from build123d import *

# Parameters (mm, degrees)
F1_DEPTH = 6
F2_D     = 12.5
F3_D     = 5
F4_D     = 5
F5_D     = 5
F6_D     = 5
F7_R     = 5
F8_D     = 8
F8_DEPTH = 20
F8_TIP   = 2.4034424761
F9_D     = 6


with BuildPart() as f1:
    # F0 (on Front) → F1 (new body)
    with BuildSketch(Plane.XZ):
        Polygon((0, 27), (0, -27), (13, -27), (40, -27), (40, 55), (26, 55), (26, 73), (0, 73), align=None)
    extrude(amount=F1_DEPTH)

    # F2 (through all)
    with Locations(Plane(origin=(0, 0, 0), x_dir=(1, 0, 0), z_dir=(0, 1, 0))):
        with Locations((13, 7)):
            Hole(F2_D / 2)

    # F3 (through all)
    with Locations(Plane(origin=(0, 0, 0), x_dir=(1, 0, 0), z_dir=(0, 1, 0))):
        with Locations((34, 21), (34, -32)):
            Hole(F3_D / 2)

    # F4 (through all)
    with Locations(Plane(origin=(0, 0, 0), x_dir=(1, 0, 0), z_dir=(0, 1, 0))):
        with Locations((5, -32), (21, -32)):
            Hole(F4_D / 2)

    # F5 (through all)
    with Locations(Plane(origin=(0, 0, 0), x_dir=(1, 0, 0), z_dir=(0, 1, 0))):
        with Locations((5, 21), (5, -9)):
            Hole(F5_D / 2)

    # F6 (through all)
    with Locations(Plane(origin=(0, 0, 0), x_dir=(1, 0, 0), z_dir=(0, 1, 0))):
        with Locations((5, -68), (21, -68)):
            Hole(F6_D / 2)

    # F7
    f7_edges = [f1.edges().sort_by_distance(p)[0] for p in [
        (26, -3, 73),
        (0, -3, 73),
        (40, -3, 55),
        (26, -3, 55),
        (40, -3, -27),
        (0, -3, -27),
    ]]
    fillet(f7_edges, radius=F7_R)

    # F8
    with Locations(Plane(origin=(0, 0, 0), x_dir=(1, 0, 0), z_dir=(0, 1, 0))):
        with Locations((13, -55.5)):
            Hole(F8_D / 2, depth=F8_DEPTH)
            with Locations((0, 0, -(F8_DEPTH + F8_TIP / 2))):  # 118° drill point
                Cone(0, F8_D / 2, F8_TIP, mode=Mode.SUBTRACT)

    # F9 (through all)
    with Locations(Plane(origin=(0, 0, 0), x_dir=(1, 0, 0), z_dir=(0, 1, 0))):
        with Locations((34, -49)):
            Hole(F9_D / 2)


solid = f1.part
Could you check a few things on this model? Use its own coordinates, in mm. Give positions to 0.01 mm unless a question says otherwise; leave off trailing zeros. Order: outer loops, then holes, each group sorted by start corner. A loop starts at its lowest first (then second) coordinate and runs counter-clockwise, first axis right, second up. Notation, with made-up numbers: (33.25, 17) - (57.25, 17) arc R29 ccw to (57.25, 45) - close; hole circle Ø3 at (-5, -12). An arc over 180 degrees is marked (long way). Return JSON: item names as keys, results as strings. Group by question number.
Q1. Please list where these lines run through material, in increasing order: line 1 along Z through (x, y) = (21, -4.55); line 2 along X through (y, z) = (-2.2, 32); line 3 along Z through (x, y) = (5, -4.3). Write a range as [from, to].
Q2. Will this pin go through, and if not, where does the flat tip stop? pin 1 Ø5 at (x, z) = (12.5, 7.5) entering from +Y.
Q3. Thinking about a two-plate mould opening in X: for faces 1 (the face through (26, -3, 64)), 2 (the face through (3.85, -3.04, 11.22)), 3 (the face through (33, -3, 55)), 4 (the face through (36.21, -3.04, 46.97)), which applies, pulls with the +X half, pulls with the -X half, needs draft (parallel to the pull), parting line crosses it, or undercut?
Q4. Suppose I cut it at A-A, the plane x = 13. Please give me the cut outline in (y, z), and give its area (3 significant figures).
Q5. Suppose I cut it at C-C, the plane z = 9. Please give me the cut outline in (x, y).
Q6. Suppose I cut it at B-B, the plane z = 32. Please give me the cut outline in (x, y), and give its area (3 significant figures).
Q7. Suppose I cut it at D-D, the plane z = -7. Please give me the cut outline in (x, y).
Resolved:
{
 "1": {"line 1": "z = [-27, 29.5], [34.5, 65.5], [70.5, 73]", "line 2": "x = [0, 2.5], [7.5, 18.5], [23.5, 31.5], [36.5, 40]", "line 3": "z = [-27, -23.5], [-18.5, 6.5], [11.5, 29.5], [34.5, 65.5], [70.5, 73]"},
 "2": {"pin 1": "stops at y = 0"},
 "3": {"face 1": "pulls with the +X half", "face 2": "undercut", "face 3": "needs draft", "face 4": "undercut"},
 "4": {"outline": "(-6, -27) - (0, -27) - (0, -13.25) - (-6, -13.25) - close; (-6, -0.75) - (0, -0.75) - (0, 51.5) - (-6, 51.5) - close; (-6, 59.5) - (0, 59.5) - (0, 73) - (-6, 73) - close", "area": "477 mm2"},
 "5": {"outline": "(0, -6) - (2.5, -6) - (2.5, 0) - (0, 0) - close; (7.5, -6) - (40, -6) - (40, 0) - (7.5, 0) - close"},
 "6": {"outline": "(0, -6) - (2.5, -6) - (2.5, 0) - (0, 0) - close; (7.5, -6) - (18.5, -6) - (18.5, 0) - (7.5, 0) - close; (23.5, -6) - (31.5, -6) - (31.5, 0) - (23.5, 0) - close; (36.5, -6) - (40, -6) - (40, 0) - (36.5, 0) - close", "area": "150 mm2"},
 "7": {"outline": "(0, -6) - (6.75, -6) - (6.75, 0) - (0, 0) - close; (19.25, -6) - (40, -6) - (40, 0) - (19.25, 0) - close"}
}
